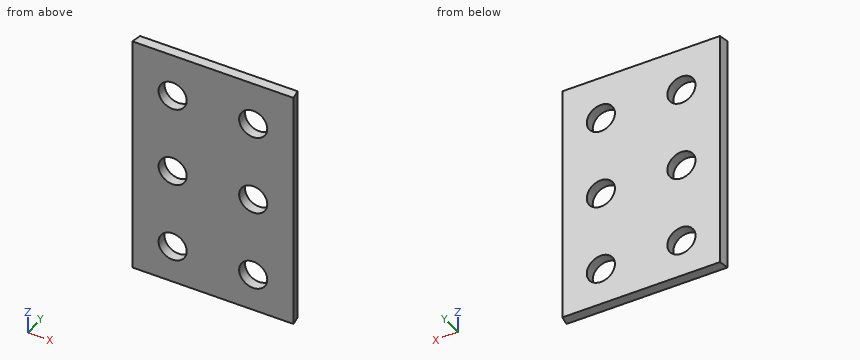
from build123d import *

# Parameters (mm, degrees)
SKETCH1_W                = 108
SKETCH1_H                = 162
SKETCH1_R                = 9.438144972
BOSS_EXTRUDE1_DEPTH      = 6.75
CUT_EXTRUDE16_DEPTH      = 500
CUT_EXTRUDE16_DEPTH_BACK = 6.75


with BuildPart() as part:
    # Sketch1 → Boss-Extrude1 (new body)
    with BuildSketch(Plane(origin=(0, 0, 0), x_dir=(1, 0, 0), z_dir=(0, 1, 0))):
        with Locations((54, -81)):
            Rectangle(SKETCH1_W, SKETCH1_H)
        with Locations(Location((27, -133.156149589, 0), (0, 0, 270))):
            Circle(SKETCH1_R, mode=Mode.SUBTRACT)
        with Locations(Location((81, -133.156149589, 0), (0, 0, 270))):
            Circle(SKETCH1_R, mode=Mode.SUBTRACT)
        with Locations(Location((81, -79.156149589, 0), (0, 0, 270))):
            Circle(SKETCH1_R, mode=Mode.SUBTRACT)
        with Locations(Location((81, -25.156149589, 0), (0, 0, 270))):
            Circle(SKETCH1_R, mode=Mode.SUBTRACT)
        with Locations(Location((27, -79.156149589, 0), (0, 0, 270))):
            Circle(SKETCH1_R, mode=Mode.SUBTRACT)
        with Locations(Location((27, -25.156149589, 0), (0, 0, 270))):
            Circle(SKETCH1_R, mode=Mode.SUBTRACT)
    extrude(amount=BOSS_EXTRUDE1_DEPTH)

    # Sketch2 → Cut-Extrude16 (cut, two sides: drawn at the far end of the back side and taken through both)
    with BuildSketch(Plane.XY.offset(-CUT_EXTRUDE16_DEPTH_BACK)):
        Polygon((0, 6.75), (0, 0), (1.19020712, 6.75), align=None)
        Polygon((108, 6.75), (108, 0), (106.80979288, 6.75), align=None)
    extrude(amount=CUT_EXTRUDE16_DEPTH + CUT_EXTRUDE16_DEPTH_BACK, mode=Mode.SUBTRACT)


solid = part.part
Work out the finished part from the listing and answer in its coordinate system (mm). Give positions to 0.01 mm unless a question says otherwise; leave off trailing zeros. Loops run counter-clockwise (first coordinate to the right, second up) from the corner with the lowest first, then second, coordinate; pieces in that order, holes last. Notation, with made-up numbers: (62.25, -27) -> (97.25, -27) arc R20 ccw to (97.25, -14) -> close; hole circle Ø1 at (-11, -7). An arc over 180 degrees is marked (long way). Use a Markdown table: item, result. Add a question column.
1. Section A-A on x = 81 is taken. Determine the outline of the cut face in (y, z), and give its area (3 significant figures).
2. Section B-B on z = 84.5 is taken. Determine the outline of the cut face in (x, y), and give its area (3 significant figures).
3. Find the intervals of material crossed by probe 1 along X at (y, z) = (0.75, 30.5); probe 2 along Z at (x, y) = (82, 2.75); probe 3 along Z at (x, y) = (31, 6.5), in increasing order.
4. Section C-C on y = 3.25 is taken. Determine the outline of the cut face in (x, z).
5. Section D-D on z = 131.5 is taken. Determine the outline of the cut face in (x, y).
Results below:
| question | item | result |
|---|---|---|
| 1 | outline | (0, 0) -> (6.75, 0) -> (6.75, 15.72) -> (0, 15.72) -> close; (0, 34.59) -> (6.75, 34.59) -> (6.75, 69.72) -> (0, 69.72) -> close; (0, 88.59) -> (6.75, 88.59) -> (6.75, 123.72) -> (0, 123.72) -> close; (0, 142.59) -> (6.75, 142.59) -> (6.75, 162) -> (0, 162) -> close |
| 1 | area | 711 mm^2 |
| 2 | outline | (0, 0) -> (19.22, 0) -> (19.22, 6.75) -> (1.19, 6.75) -> close; (34.78, 0) -> (73.22, 0) -> (73.22, 6.75) -> (34.78, 6.75) -> close; (88.78, 0) -> (108, 0) -> (106.81, 6.75) -> (88.78, 6.75) -> close |
| 2 | area | 511 mm^2 |
| 3 | probe 1 | x = 0.13 to 19.22, 34.78 to 73.22, 88.78 to 107.87 |
| 3 | probe 2 | z = 0 to 15.77, 34.54 to 69.77, 88.54 to 123.77, 142.54 to 162 |
| 3 | probe 3 | z = 0 to 16.61, 33.7 to 70.61, 87.7 to 124.61, 141.7 to 162 |
| 4 | outline | (0.57, 0) -> (107.43, 0) -> (107.43, 162) -> (0.57, 162) -> close; hole circle Ø18.88 at (27, 25.16); hole circle Ø18.88 at (27, 79.16); hole circle Ø18.88 at (27, 133.16); hole circle Ø18.88 at (81, 25.16); hole circle Ø18.88 at (81, 79.16); hole circle Ø18.88 at (81, 133.16) |
| 5 | outline | (0, 0) -> (17.71, 0) -> (17.71, 6.75) -> (1.19, 6.75) -> close; (36.29, 0) -> (71.71, 0) -> (71.71, 6.75) -> (36.29, 6.75) -> close; (90.29, 0) -> (108, 0) -> (106.81, 6.75) -> (90.29, 6.75) -> close |
